```python
from build123d import *

# Parameters (mm, degrees)
SKETCH1_R               = 52.5
SKETCH1_R_2             = 8
BOSS_EXTRUDE1_DEPTH     = 6
SKETCH2_R               = 14
BOSS_EXTRUDE2_DEPTH     = 7
CUT_EXTRUDE1_DEPTH      = 77
SKETCH4_R               = 49
CUT_EXTRUDE2_DEPTH      = 3.5
CUT_EXTRUDE2_DRAFT      = -40
FILLET1_R               = 20
MIRROR1_COPY_1_SKETCH_R = 49
MIRROR1_COPY_1_DEPTH    = 3.5
MIRROR1_COPY_1_DRAFT    = -40
SKETCH6_R               = 14
BOSS_EXTRUDE3_DEPTH     = 10.5
FILLET2_R               = 1.5
FILLET3_R               = 2


with BuildPart() as part:
    # Sketch1 → Boss-Extrude1 (new, symmetric)
    with BuildSketch(Plane(origin=(0, 0, 0), x_dir=(1, 0, 0), z_dir=(0, 1, 0))):
        with Locations(Location((0, 0, 0), (0, 0, 270))):
            Circle(SKETCH1_R)
        with Locations(Location((0, 30, 0), (0, 0, 270))):
            Circle(SKETCH1_R_2, mode=Mode.SUBTRACT)
        with Locations(Location((25.980762114, 15, 0), (0, 0, 270))):
            Circle(SKETCH1_R_2, mode=Mode.SUBTRACT)
        with Locations(Location((25.980762114, -15, 0), (0, 0, 270))):
            Circle(SKETCH1_R_2, mode=Mode.SUBTRACT)
        with Locations(Location((0, -30, 0), (0, 0, 270))):
            Circle(SKETCH1_R_2, mode=Mode.SUBTRACT)
        with Locations(Location((-25.980762114, -15, 0), (0, 0, 270))):
            Circle(SKETCH1_R_2, mode=Mode.SUBTRACT)
        with Locations(Location((-25.980762114, 15, 0), (0, 0, 270))):
            Circle(SKETCH1_R_2, mode=Mode.SUBTRACT)
    extrude(amount=BOSS_EXTRUDE1_DEPTH, both=True)

    # Sketch2 → Boss-Extrude2 (add)
    with BuildSketch(Plane.XZ.offset(6)):
        with Locations(Location((0, 0, 0), (0, 0, 270))):
            Circle(SKETCH2_R)
    extrude(amount=BOSS_EXTRUDE2_DEPTH)

    # Sketch3 → Cut-Extrude1 (cut)
    with BuildSketch(Plane.XZ.offset(13)):
        with BuildLine():
            Line((-8.4, 2.5), (-8.4, -2.5))
            Line((-8.4, -2.5), (-6.538348415, -2.5))
            ThreePointArc((-6.538348415, -2.5), (7, 0), (-6.538348415, 2.5))
            Line((-6.538348415, 2.5), (-8.4, 2.5))
        make_face()
    extrude(amount=-CUT_EXTRUDE1_DEPTH, mode=Mode.SUBTRACT)


with BuildPart() as cut_extrude2_tool:
    # Sketch4 → Cut-Extrude2 (with draft: the straight prism first)
    with BuildSketch(Plane(origin=(0, 6, 0), x_dir=(1, 0, 0), z_dir=(0, 1, 0))):
        Circle(SKETCH4_R)
    extrude(amount=-CUT_EXTRUDE2_DEPTH)
    # Cut-Extrude2: the draft: its side faces are tilted about the plane it starts from
    cut_extrude2_sides = [cut_extrude2_tool.faces().sort_by_distance(p)[0] for p in [
        (-49, 4.25, 0),
    ]]
    draft(cut_extrude2_sides, Plane(origin=(0, 6, 0), x_dir=(1, 0, 0), z_dir=(0, 1, 0)), CUT_EXTRUDE2_DRAFT)


with BuildPart() as part_1:
    add(part.part)

    # Cut-Extrude2: cut by cut_extrude2_tool
    add(cut_extrude2_tool.part, mode=Mode.SUBTRACT)

    # Fillet1
    # the kernel refuses this fillet: 20 mm, written as the material it adds along each edge
    with BuildSketch(Plane(origin=(0, 2.5, 0), x_dir=(1, 0, 0), z_dir=(0, 0, 1))) as fillet1_piece_1_section:
        with BuildLine():
            CenterArc((37.697345445, 20), FILLET1_R, 270, 34.41150867)
            Line((37.697345445, 0), (37.697345445, -0.4))
            Line((37.697345445, -0.4), (46.063151291, -0.4))
            Line((46.063151291, -0.4), (46.369569068, -0.257115044))
            ThreePointArc((46.369569068, -0.257115044), (47.837993423, 1.492884956), (49.226053091, 3.17))
            Line((49.226053091, 3.17), (49, 3.5))
        make_face()
    fillet1_piece_1 = revolve(axis=Axis((0, 2.5, 0), (0, 1, 0)), mode=Mode.PRIVATE)
    fillet1_piece_1 = fillet1_piece_1 - Plane(origin=(-25.980762114, 3.249062711, 15), x_dir=(0, 0, 1), z_dir=(0, -1, 0)) * Cylinder(8, 197, mode=Mode.PRIVATE)
    fillet1_piece_1 = fillet1_piece_1 - Plane(origin=(0, 3.249062711, 30), x_dir=(0, 0, 1), z_dir=(0, -1, 0)) * Cylinder(8, 197, mode=Mode.PRIVATE)
    fillet1_piece_1 = fillet1_piece_1 - Plane(origin=(25.980762114, 3.249062711, 15), x_dir=(0, 0, 1), z_dir=(0, -1, 0)) * Cylinder(8, 197, mode=Mode.PRIVATE)
    fillet1_piece_1 = fillet1_piece_1 - Plane(origin=(-25.980762114, 3.249062711, -15), x_dir=(0, 0, 1), z_dir=(0, -1, 0)) * Cylinder(8, 197, mode=Mode.PRIVATE)
    fillet1_piece_1 = fillet1_piece_1 - Plane(origin=(0, 3.249062711, -30), x_dir=(0, 0, 1), z_dir=(0, -1, 0)) * Cylinder(8, 197, mode=Mode.PRIVATE)
    fillet1_piece_1 = fillet1_piece_1 - Plane(origin=(25.980762114, 3.249062711, -15), x_dir=(0, 0, 1), z_dir=(0, -1, 0)) * Cylinder(8, 197, mode=Mode.PRIVATE)
    add(fillet1_piece_1)


with BuildPart() as mirror1_copy_1_tool:
    # Mirror1 copy 1 sketch → Mirror1 copy 1 (with draft: the straight prism first)
    with BuildSketch(Plane.XZ.offset(6)):
        Circle(MIRROR1_COPY_1_SKETCH_R)
    extrude(amount=-MIRROR1_COPY_1_DEPTH)
    # Mirror1 copy 1: the draft: its side faces are tilted about the plane it starts from
    mirror1_copy_1_sides = [mirror1_copy_1_tool.faces().sort_by_distance(p)[0] for p in [
        (-49, -4.25, 0),
    ]]
    draft(mirror1_copy_1_sides, Plane.XZ.offset(6), MIRROR1_COPY_1_DRAFT)


with BuildPart() as part_2:
    add(part_1.part)

    # Mirror1 copy 1: cut by mirror1_copy_1_tool
    add(mirror1_copy_1_tool.part, mode=Mode.SUBTRACT)

    # Sketch5 → Cut-Revolve1 (revolve, cut)
    with BuildSketch(Plane.XY, mode=Mode.PRIVATE) as cut_revolve1_sk:
        Polygon((52.5, 3.5), (52.5, -3.5), (46.5, -1.316178594), (46.5, 1.316178594), align=None)
    revolve(cut_revolve1_sk.sketch.rotate(Axis((0, 0, 0), (0, 1, 0)), 90), axis=Axis((0, 0, 0), (0, 1, 0)), mode=Mode.SUBTRACT)

    # Sketch6 → Boss-Extrude3 (add)
    with BuildSketch(Plane.XZ.offset(13)):
        with Locations(Location((0, 0, 0), (0, 0, 270))):
            Circle(SKETCH6_R)
        with BuildLine():
            Line((-8.4, 2.5), (-8.4, -2.5))
            Line((-8.4, -2.5), (-6.538348415, -2.5))
            ThreePointArc((-6.538348415, -2.5), (7, 0), (-6.538348415, 2.5))
            Line((-6.538348415, 2.5), (-8.4, 2.5))
        make_face(mode=Mode.SUBTRACT)
    extrude(amount=-BOSS_EXTRUDE3_DEPTH)

    # Fillet2
    fillet2_edges = [part_2.edges().sort_by_distance(p)[0] for p in [
        (0, -13, 14),
    ]]
    fillet(fillet2_edges, radius=FILLET2_R)

    # Fillet3
    fillet3_edges = [part_2.edges().sort_by_distance(p)[0] for p in [
        (0, -2.5, 14),
    ]]
    fillet(fillet3_edges, radius=FILLET3_R)


solid = part_2.part
```
The model under review builds one solid part; all positions refer to its coordinate system, in mm. A direction names the side the tool comes from. Give positions to 0.01 mm unless a question says otherwise; leave off trailing zeros. Write each loop counter-clockwise with the first axis right and the second up, starting at its lowest first coordinate (ties: lowest second). Pieces come first, ordered by that corner, then holes. Notation, with made-up numbers: M -19.5,10 L 38.5,10 A27 cw 38.5,38 Z; hole C 54.5,2 d1. An arc over 180 degrees is marked long. Write item = value, one per line. Start each with the question number.
Q1. We need section B-B (x = 29). Give the number of separate pieces and of enclosed holes in the cut face, plus the area to 3 significant figures.
Q2. Clearance check with flat-ended pins moving along their axes: pin 1 (2 mm diameter, centred on x = -7.5, y = -5, fed in from +Z); pin 2 (21 mm diameter, centred on x = -25.98, z = -15, fed in from -Y); pin 3 (1 mm diameter, centred on y = 0.5, z = 24.5, fed in from -X). State where each tip first meets the part, or that it passes through.
Q3. Machinability: for faces 1 (the face through (-14.08, 1.453, -44.711)), 2 (the face through (-8.4, -5, 0)), 3 (the face through (-1, 2.5, 8)), 4 (the face through (-5.4, -13, -5.4)), which of the approach directions +Z, -Z, +X, -X, +Y, -Y give a long, thin tool a straight path to every point of the face, cutting with its end or side? Answer none if there is none.
Q4. For line 1 (Y direction, x = 27, z = -38); line 2 (Y direction, x = 24, z = 2); line 3 (Z direction, x = -23, y = 4.5), list the stretches that pass through material, from the lowest coordinate up.
Q5. We need section A-A (y = -8.25). State the section outline as (x, z) points, plus the area to 3 significant figures.
Q6. Mouldability with a two-part tool opening along Y and no side actions: class faces 5 (the face through (24, 6, -43)), 6 (the face through (20, -2.5, 1)), 7 (the face through (41.51, -1.42, -21.59)), 8 (the face through (15.77, 4.768, 50.076)) as released by +Y, released by -Y, zero draft, split by the parting line, or undercut.
Result set:
q1.separate_pieces = 3
q1.enclosed_holes = 0
q1.area = 324 mm2
q2.pin_1 = 52.1
q2.pin_2 = -2.5
q2.pin_3 = -39.83
q3.face_1 = none
q3.face_2 = +Y, -Y
q3.face_3 = +Y
q3.face_4 = +Z, -Z, +X, -X, -Y
q4.line_1 = -3.16 to -1.36, 1.36 to 4.6
q4.line_2 = -2.5 to 2.5
q4.line_3 = -47.19 to -40.32, 40.32 to 47.19
q5.outline = C 0,0 d28; hole M -8.4,-2.5 L -6.54,-2.5 A7 ccw long -6.54,2.5 L -8.4,2.5 Z
q5.area = 454 mm2
q6.face_5 = released by +Y
q6.face_6 = released by -Y
q6.face_7 = undercut
q6.face_8 = zero draft
